Part model, mm, in its own coordinate system. A direction names the side the tool comes from. Give positions to 0.01 mm unless a question says otherwise; leave off trailing zeros. Order: outer loops, then holes, each group sorted by start corner. A loop starts at its lowest first (then second) coordinate and runs counter-clockwise, first axis right, second up. Notation, with made-up numbers: (63.5, 55.5) -> (75.5, 55.5) arc R27 cw to (75.5, 93.5) -> close; hole circle Ø7 at (0.25, 26). An arc over 180 degrees is marked (long way). Write item = value, one per line. Start each with the question number.
Item 1: Band-saw the part on C-C on z = 27. Write the cut outline in (x, y), plus the area to 3 significant figures.
Item 2: Band-saw the part on B-B on x = 4. Write the cut outline in (y, z), plus the area to 3 significant figures.
Item 3: Pull direction Z, two halves, no side cores. Call faces 6 (the face through (12, -161, 127)), 7 (the face through (5.92, -157.59, 133.04)), 8 (the face through (-1, 2, 230)): +Z half, -Z half, draft (parallel to the pull), parting line (faces both ways), or undercut.
Item 4: Band-saw the part on D-D on x = -19. Write the cut outline in (y, z), plus the area to 3 significant figures.
Item 5: Flat gauge pin, fed straight in: P1, Ø2, axis at x = -58.5, z = 110.5, coming from the -Y side. Where does the tip first touch, or does it go through?
Item 6: Drill centre lines: line 1 along Y through (x, z) = (-73.5, 177); line 2 along Z through (x, y) = (-24, -144). Where is each one in solid material? Low to high.
Item 7: Tool access for faces 1 (the face through (5.92, -149.25, 170.17)), 2 (the face through (0, -161, 127)), 3 (the face through (-5.83, -154.82, 0.74)), 4 (the face through (5.92, -165.47, 135.56)), 5 (the face through (6, -155, 84)): list every direction of +Z, -Z, +X, -X, +Y, -Y with a clear straight run to the whole face (end or side of a thin tool).
Item 8: Band-saw the part on A-A on z = 116. Write the cut outline in (x, y).
```python
from build123d import *

# Parameters (mm, degrees)
F0_W     = 190
F0_H     = 285
F1_DEPTH = 230
F2_R     = 26.9
F3_DEPTH = 25
F5_DEPTH = 12


with BuildPart() as f1:
    # F0 (on Top) → F1 (new body)
    with BuildSketch(Plane.XY):
        Rectangle(F0_W, F0_H)
    extrude(amount=F1_DEPTH)

    # F2 (on face) → F3 (join)
    with BuildSketch(Plane.XZ.offset(142.5)):
        with Locations((0, 27)):
            Circle(F2_R)
    extrude(amount=F3_DEPTH)

    # F4 (on Right) → F5 (join)
    with BuildSketch(Plane.YZ):
        Polygon((-142.5, 171.776368), (-142.5, 180), (-163.5, 175), (-167.5, 95), (-142.5, 73), (-142.5, 83.656529), (-159.317222, 98.455684), (-155.809636, 168.607407), align=None)
    extrude(amount=F5_DEPTH)


solid = f1.part
```
Values found:
q1.outline = (-95, -142.5) -> (-26.9, -142.5) -> (-26.9, -167.5) -> (26.9, -167.5) -> (26.9, -142.5) -> (95, -142.5) -> (95, 142.5) -> (-95, 142.5) -> close
q1.area = 55,500 mm^2
q2.outline = (-167.5, 0.4) -> (-142.5, 0.4) -> (-142.5, 0) -> (142.5, 0) -> (142.5, 230) -> (-142.5, 230) -> (-142.5, 180) -> (-163.5, 175) -> (-167.5, 95) -> (-142.5, 73) -> (-142.5, 53.6) -> (-167.5, 53.6) -> close; hole (-159.32, 98.46) -> (-142.5, 83.66) -> (-142.5, 171.78) -> (-155.81, 168.61) -> close
q2.area = 67,800 mm^2
q3.face_6 = draft
q3.face_7 = undercut
q3.face_8 = +Z half
q4.outline = (-167.5, 7.96) -> (-142.5, 7.96) -> (-142.5, 0) -> (142.5, 0) -> (142.5, 230) -> (-142.5, 230) -> (-142.5, 46.04) -> (-167.5, 46.04) -> close
q4.area = 66,500 mm^2
q5.P1 = -142.5
q6.line_1 = -142.5 to 142.5
q6.line_2 = 14.85 to 39.15
q7.face_1 = +X, -X
q7.face_2 = +Z, -X, -Y
q7.face_3 = -Y
q7.face_4 = +Z, +X, -X, -Y
q7.face_5 = +X, -X, -Y
q8.outline = (-95, -142.5) -> (95, -142.5) -> (95, 142.5) -> (-95, 142.5) -> close; (0, -166.45) -> (12, -166.45) -> (12, -158.44) -> (0, -158.44) -> close
